from build123d import *

# Parameters (mm, degrees)
BOSS_EXTRUDE1_DEPTH = 63.5
SKETCH10_R          = 2.5019
CUT_EXTRUDE3_DEPTH  = 12.7
BOSS_EXTRUDE2_START = -60.325
SKETCH12_R          = 12.5
BOSS_EXTRUDE2_DEPTH = 3.175
SKETCH14_R          = 1.5875
CUT_EXTRUDE4_DEPTH  = 6.35
CUT_EXTRUDE5_REACH  = 107.322
SKETCH15_R          = 10.668


with BuildPart() as part:
    # Sketch1 → Boss-Extrude1 (new body)
    with BuildSketch(Plane.XY):
        with BuildLine():
            Line((37.577733998, 36.783983953), (37.577733998, -36.783983998))
            ThreePointArc((37.577733998, -36.783983998), (37.345250005, -37.345250005), (36.783983998, -37.577733998))
            Line((36.783983998, -37.577733998), (-36.783983953, -37.577733998))
            ThreePointArc((-36.783983953, -37.577733998), (-37.34524996, -37.345250005), (-37.577733953, -36.783983998))
            Line((-37.577733953, -36.783983998), (-37.577733953, 36.783983953))
            ThreePointArc((-37.577733953, 36.783983953), (-37.34524996, 37.34524996), (-36.783983953, 37.577733953))
            Line((-36.783983953, 37.577733953), (36.783983998, 37.577733953))
            ThreePointArc((36.783983998, 37.577733953), (37.345250005, 37.34524996), (37.577733998, 36.783983953))
        make_face()
        with BuildLine():
            Line((-16.61571496, 30.582545515), (16.61571496, 30.582545515))
            ThreePointArc((16.61571496, 30.582545515), (26.491755557, 26.491755557), (30.582545515, 16.61571496))
            Line((30.582545515, 16.61571496), (30.582545515, -16.61571496))
            ThreePointArc((30.582545515, -16.61571496), (26.491755557, -26.491755557), (16.61571496, -30.582545515))
            Line((16.61571496, -30.582545515), (-16.61571496, -30.582545515))
            ThreePointArc((-16.61571496, -30.582545515), (-26.491755557, -26.491755557), (-30.582545515, -16.61571496))
            Line((-30.582545515, -16.61571496), (-30.582545515, 16.61571496))
            ThreePointArc((-30.582545515, 16.61571496), (-26.491755557, 26.491755557), (-16.61571496, 30.582545515))
        make_face(mode=Mode.SUBTRACT)
    extrude(amount=-BOSS_EXTRUDE1_DEPTH)

    # Sketch10 → Cut-Extrude3 (cut)
    with BuildSketch(Plane.XY):
        with Locations((33.488333998, 33.488333998)):
            Circle(SKETCH10_R)
        with Locations((33.488333998, -33.488333998)):
            Circle(SKETCH10_R)
        with Locations((-33.488333998, -33.488333998)):
            Circle(SKETCH10_R)
        with Locations((-33.488333998, 33.488333998)):
            Circle(SKETCH10_R)
    extrude(amount=-CUT_EXTRUDE3_DEPTH, mode=Mode.SUBTRACT)

    # Sketch12 → Boss-Extrude2 (add)
    with BuildSketch(Plane.XY.offset(BOSS_EXTRUDE2_START)):
        with BuildLine():
            Line((37.577733998, 36.783983953), (37.577733998, -36.783983998))
            ThreePointArc((37.577733998, -36.783983998), (37.345250005, -37.345250005), (36.783983998, -37.577733998))
            Line((36.783983998, -37.577733998), (-36.783983953, -37.577733998))
            ThreePointArc((-36.783983953, -37.577733998), (-37.34524996, -37.345250005), (-37.577733953, -36.783983998))
            Line((-37.577733953, -36.783983998), (-37.577733953, 36.783983953))
            ThreePointArc((-37.577733953, 36.783983953), (-37.34524996, 37.34524996), (-36.783983953, 37.577733953))
            Line((-36.783983953, 37.577733953), (36.783983998, 37.577733953))
            ThreePointArc((36.783983998, 37.577733953), (37.345250005, 37.34524996), (37.577733998, 36.783983953))
        make_face()
        Circle(SKETCH12_R, mode=Mode.SUBTRACT)
    extrude(amount=-BOSS_EXTRUDE2_DEPTH)

    # Sketch14 → Cut-Extrude4 (cut)
    with BuildSketch(Plane(origin=(37.577733998, 0, 0), x_dir=(0, 0, -1), z_dir=(1, 0, 0))):
        with Locations(Location((50.8, 33.005733953, 0), (0, 0, 90))):
            Circle(SKETCH14_R)
        with Locations(Location((50.8, -33.005733998, 0), (0, 0, 90))):
            Circle(SKETCH14_R)
    extrude(amount=-CUT_EXTRUDE4_DEPTH, mode=Mode.SUBTRACT)

    # Sketch15 → Cut-Extrude5 (cut, up to next)
    with BuildSketch(Plane.XZ.offset(-37.577733953), mode=Mode.PRIVATE) as cut_extrude5_sk1:
        with Locations(Location((0, -31.75, 0), (0, 0, 180))):
            Circle(SKETCH15_R)
    cut_extrude5_tool1 = extrude(cut_extrude5_sk1.sketch, amount=CUT_EXTRUDE5_REACH, mode=Mode.PRIVATE) & part.part
    add(cut_extrude5_tool1.solids().sort_by_distance((0, 37.577734, -31.75))[0], mode=Mode.SUBTRACT)


solid = part.part
CAD build for the part. Positions are in the model's coordinates, mm. A direction names the side the tool comes from. Round coordinates to 2 decimals unless told otherwise and drop trailing zeros. Order: outer loops, then holes, each group sorted by start corner. A loop starts at its lowest first (then second) coordinate and runs counter-clockwise, first axis right, second up. Notation, with made-up numbers: M -30.75,-13.75 L -20.75,-13.75 A4 ccw -20.75,-7.75 Z; hole C 48,-13 d10. An arc over 180 degrees is marked long. Use one line per item in the form item = value.
Q1. Saw through at C-C on z = -15.5. Give the cut face in (x, y), then the cut area to 3 significant figures.
Recorded:
outline = M -37.58,-36.78 A0.79 ccw -36.78,-37.58 L 36.78,-37.58 A0.79 ccw 37.58,-36.78 L 37.58,36.78 A0.79 ccw 36.78,37.58 L -36.78,37.58 A0.79 ccw -37.58,36.78 Z; hole M -30.58,-16.62 A13.97 ccw -16.62,-30.58 L 16.62,-30.58 A13.97 ccw 30.58,-16.62 L 30.58,16.62 A13.97 ccw 16.62,30.58 L -16.62,30.58 A13.97 ccw -30.58,16.62 Z
area = 2,070 mm^2
Q2. Which spindle directions (+Z, -Z, +X, -X, +Y, -Y) get a long thin tool onto all of the face, cutting with end or side? Do faces 1 (the cylindrical face through (2.313, 34.129, -21.336)), 2 (the cylindrical face through (-35.332, -31.797, -6.261)), 3 (the flat face through (31.228, -33, -51)). Say none if no direction does.
Recorded:
face_1 = +Y
face_2 = +Z
face_3 = +X
Q3. Probe L1, parallel to X at y = 15.5, z = -32; L2, parallel to Y at x = 0, z = -62. List the from-to ranges inside material, lowest first.
Recorded:
L1 = -37.58 to -30.58, 30.58 to 37.58
L2 = -37.58 to -12.5, 12.5 to 37.58
Q4. Saw through at A-A on y = 0. Give the cut face in (x, z) (3 decimals).
Recorded:
outline = M -37.578,-63.5 L -12.5,-63.5 L -12.5,-60.325 L -30.583,-60.325 L -30.583,0 L -37.578,0 Z; M 12.5,-63.5 L 37.578,-63.5 L 37.578,0 L 30.583,0 L 30.583,-60.325 L 12.5,-60.325 Z
Q5. Saw through at D-D on z = -31.75. Give the cut face in (x, y), then the cut area to 3 significant figures.
Recorded:
outline = M -37.58,-36.78 A0.79 ccw -36.78,-37.58 L 36.78,-37.58 A0.79 ccw 37.58,-36.78 L 37.58,36.78 A0.79 ccw 36.78,37.58 L 10.67,37.58 L 10.67,30.58 L 16.62,30.58 A13.97 cw 30.58,16.62 L 30.58,-16.62 A13.97 cw 16.62,-30.58 L -16.62,-30.58 A13.97 cw -30.58,-16.62 L -30.58,16.62 A13.97 cw -16.62,30.58 L -10.67,30.58 L -10.67,37.58 L -36.78,37.58 A0.79 ccw -37.58,36.78 Z
area = 1,920 mm^2
Q6. Flat gauge pins, fed straight in: P1, Ø19, axis at x = 0, z = -31.75, coming from the +Y side; P2, Ø1, axis at y = 33.5, z = -50.5, coming from the +X side; P3, Ø4, axis at x = 28, y = 1.5, coming from the +Z side (3 decimals); P4, Ø5.5, axis at x = -32.5, y = -33, coming from the +Z side. Where does each tip first touch, or does it go through?
Recorded:
P1 = -30.58
P2 = 31.23
P3 = -60.325
P4 = 0
Q7. Saw through at B-B on x = -9. Give the cut face in (y, z) (3 decimals).
Recorded:
outline = M -37.578,-63.5 L -8.675,-63.5 L -8.675,-60.325 L -30.583,-60.325 L -30.583,0 L -37.578,0 Z; M 8.675,-63.5 L 37.578,-63.5 L 37.578,-37.478 L 30.583,-37.478 L 30.583,-60.325 L 8.675,-60.325 Z; M 30.583,-26.022 L 37.578,-26.022 L 37.578,0 L 30.583,0 Z
Q8. Two-plate mould, pull along X, no slides. Class faces 4 (the cylindrical face through (26.6, -26.38, -29.74)), 5 (the flat face through (9, 9, -63.5)), 6 (the flat face through (31.228, 33, -51)): +X half, -X half, draft (parallel to the pull), parting line (faces both ways), or undercut.
Recorded:
face_4 = undercut
face_5 = draft
face_6 = +X half
